Read the model definition and answer for the solid it produces. Units are mm, in the model's axes. A direction names the side the tool comes from. Give positions to 0.01 mm unless a question says otherwise; leave off trailing zeros. Write each loop counter-clockwise with the first axis right and the second up, starting at its lowest first coordinate (ties: lowest second). Pieces come first, ordered by that corner, then holes. Notation, with made-up numbers: M 31.5,7 L 45.5,7 A27 ccw 45.5,40 Z; hole C 15.5,-10 d1. An arc over 180 degrees is marked long. Use a Markdown table: item, result. Add a question column.
Item 1: A cutting plane is placed at C-C on x = 20.5. Determine the outline of the cut face in (y, z), then the cut area to 3 significant figures.
Item 2: A cutting plane is placed at A-A on x = 0. Determine the outline of the cut face in (y, z), then the cut area to 3 significant figures.
Item 3: A cutting plane is placed at B-B on z = -4. Determine the outline of the cut face in (x, y), then the cut area to 3 significant figures.
Item 4: A cutting plane is placed at D-D on x = -15. Determine the outline of the cut face in (y, z), then the cut area to 3 significant figures.
Item 5: Consider probe 1 along Z at (x, y) = (-11.5, -37); probe 2 along X at (y, z) = (2.5, 0.25); probe 3 along X at (y, z) = (5.5, -1). Determine where each line is inside the solid, lowest interval first. Write a range as [from, to].
Item 6: For faces 1 (the flat face through (-14, -33, -0.254)), 2 (the flat face through (14, -33, 0)), 3 (the flat face through (-14, -33, 0)), 4 (the flat face through (14, -33, -0.254)), determine the directions among +Z, -Z, +X, -X, +Y, -Y from which every point of the face is accessible in a straight line to the end or side of a thin tool.
Item 7: Given P1, Ø8, axis at x = -18.5, y = -27, coming from the -Z side; P2, Ø2, axis at x = 5, y = 4.5, coming from the -Z side; P3, Ø12.5, axis at x = 17.5, y = -32, coming from the +Z side; P4, Ø2, axis at x = 8.5, y = 10, coming from the -Z side, each flat-ended and moving along its own axis, determine where each tip first touches the part or whether it passes through.
from build123d import *

# Parameters (mm, degrees)
F0_R     = 7.810875
F1_DEPTH = 74.422
F2_R     = 5.797625
F3_DEPTH = 21.59
F4_R     = 23.677635
F5_DEPTH = 0.254


with BuildPart() as f1:
    # F0 (on Front) → F1 (new body)
    with BuildSketch(Plane.XZ):
        Circle(F0_R)
    extrude(amount=F1_DEPTH)

    # F2 (on Front) → F3 (join)
    with BuildSketch(Plane.XZ):
        Circle(F2_R)
    extrude(amount=-F3_DEPTH)

    # F4 (on Top) → F5 (join)
    with BuildSketch(Plane.XY):
        with Locations((0, -33.121504)):
            Circle(F4_R)
    extrude(amount=-F5_DEPTH)


solid = f1.part
Filled in:
| question | item | result |
|---|---|---|
| 1 | outline | M -44.97,-0.25 L -21.27,-0.25 L -21.27,0 L -44.97,0 Z |
| 1 | area | 6.02 mm² |
| 2 | outline | M -74.42,-7.81 L 0,-7.81 L 0,-5.8 L 21.59,-5.8 L 21.59,5.8 L 0,5.8 L 0,7.81 L -74.42,7.81 Z |
| 2 | area | 1,410 mm² |
| 3 | outline | M -6.71,-74.42 L 6.71,-74.42 L 6.71,0 L 4.2,0 L 4.2,21.59 L -4.2,21.59 L -4.2,0 L -6.71,0 Z |
| 3 | area | 1,180 mm² |
| 4 | outline | M -51.44,-0.25 L -14.8,-0.25 L -14.8,0 L -51.44,0 Z |
| 4 | area | 9.31 mm² |
| 5 | probe 1 | [-0.25, 0] |
| 5 | probe 2 | [-5.79, 5.79] |
| 5 | probe 3 | [-5.71, 5.71] |
| 6 | face 1 | -Z, -X, +Y, -Y |
| 6 | face 2 | +Z, +X, +Y, -Y |
| 6 | face 3 | +Z, -X, +Y, -Y |
| 6 | face 4 | -Z, +X, +Y, -Y |
| 7 | P1 | z = -0.25 |
| 7 | P2 | z = -4.2 |
| 7 | P3 | z = 0 |
| 7 | P4 | through |
